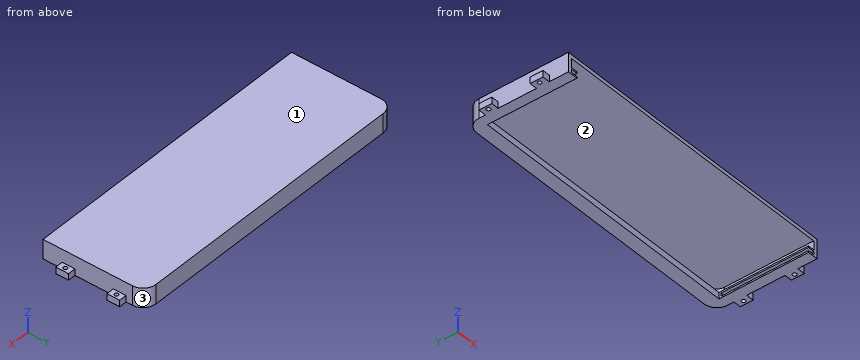
```python
from build123d import *

# Parameters (mm, degrees)
BOSS_EXTRU_1_DEPTH      = 15
COQUE1_T                = -3
ESQUISSE3_W             = 228
ESQUISSE3_H             = 3
ENL_V_MAT_EXTRU_2_DEPTH = 12
BOSS_EXTRU_3_DEPTH      = 5
BOSS_EXTRU_4_DEPTH      = 5
ESQUISSE2_W             = 6
ESQUISSE2_H             = 10
ESQUISSE2_R             = 1.5
BOSS_EXTRU_6_DEPTH      = 5


with BuildPart() as part:
    # Esquisse1 → Boss.-Extru.1 (new body)
    with BuildSketch(Plane.XY):
        with BuildLine():
            Line((-107, 40), (107, 40))
            ThreePointArc((107, 40), (114.071067812, 37.071067812), (117, 30))
            Line((117, 30), (117, -40))
            Line((117, -40), (-117, -40))
            Line((-117, -40), (-117, 30))
            ThreePointArc((-117, 30), (-114.071067812, 37.071067812), (-107, 40))
        make_face()
    extrude(amount=BOSS_EXTRU_1_DEPTH)

    # Coque1
    coque1_openings = [part.faces().sort_by_distance(p)[0] for p in [
        (0, -0.086787891, 0),
    ]]
    offset(amount=COQUE1_T, openings=coque1_openings, kind=Kind.INTERSECTION)

    # Esquisse3 → Enlèv. mat.-Extru.2 (cut)
    with BuildSketch(Plane(origin=(0, 0, 0), x_dir=(-1, 0, 0), z_dir=(0, 0, -1))):
        with Locations((0, -38.5)):
            Rectangle(ESQUISSE3_W, ESQUISSE3_H)
    extrude(amount=-ENL_V_MAT_EXTRU_2_DEPTH, mode=Mode.SUBTRACT)

    # Esquisse4 → Boss.-Extru.3 (add)
    with BuildSketch(Plane.ZY.offset(-114)):
        Polygon((0, -40), (0, 30), (5, 30), (5, -40), (3.75, -40), (3.75, 28.5), (1.25, 28.5), (1.25, -40), align=None)
    boss_extru_3 = extrude(amount=BOSS_EXTRU_3_DEPTH)

    # Symétrie1: Boss.-Extru.3 across plane
    add(boss_extru_3.mirror(Plane(origin=(0, 0, 0), x_dir=(0, 0, 1), z_dir=(1, 0, 0))))

    # Esquisse5 → Boss.-Extru.4 (add)
    with BuildSketch(Plane(origin=(0, 0, 0), x_dir=(-1, 0, 0), z_dir=(0, 0, -1))):
        with BuildLine():
            Line((-107, 37), (107, 37))
            ThreePointArc((107, 37), (111.949747468, 34.949747468), (114, 30))
            Line((114, 30), (-114, 30))
            ThreePointArc((-114, 30), (-111.949747468, 34.949747468), (-107, 37))
        make_face()
    extrude(amount=-BOSS_EXTRU_4_DEPTH)

    # Esquisse2 → Boss.-Extru.6 (add)
    # profile 1 of 4: a face of its own
    with BuildSketch(Plane(origin=(0, 0, 0), x_dir=(-1, 0, 0), z_dir=(0, 0, -1))):
        with Locations((-120, -20)):
            Rectangle(ESQUISSE2_W, ESQUISSE2_H)
        with Locations((-120, -20)):
            Circle(ESQUISSE2_R, mode=Mode.SUBTRACT)
    # profile 2 of 4: a face of its own
    with BuildSketch(Plane(origin=(0, 0, 0), x_dir=(-1, 0, 0), z_dir=(0, 0, -1))):
        with Locations((-120, 20)):
            Rectangle(ESQUISSE2_W, ESQUISSE2_H)
        with Locations((-120, 20)):
            Circle(ESQUISSE2_R, mode=Mode.SUBTRACT)
    # profile 3 of 4: a face of its own
    with BuildSketch(Plane(origin=(0, 0, 0), x_dir=(-1, 0, 0), z_dir=(0, 0, -1))):
        with Locations((120, 20)):
            Rectangle(ESQUISSE2_W, ESQUISSE2_H)
        with Locations((120, 20)):
            Circle(ESQUISSE2_R, mode=Mode.SUBTRACT)
    # profile 4 of 4: a face of its own
    with BuildSketch(Plane(origin=(0, 0, 0), x_dir=(-1, 0, 0), z_dir=(0, 0, -1))):
        with Locations((120, -20)):
            Rectangle(ESQUISSE2_W, ESQUISSE2_H)
        with Locations((120, -20)):
            Circle(ESQUISSE2_R, mode=Mode.SUBTRACT)
    extrude(amount=-BOSS_EXTRU_6_DEPTH)


solid = part.part
```
The listing builds one solid part. Answer for the finished solid, in the listing's coordinates (mm). Face numbers are marked on the shaded views. Coordinates: 2 decimals unless noted, no trailing zeros. Write each loop counter-clockwise with the first axis right and the second up, starting at its lowest first coordinate (ties: lowest second). Pieces come first, ordered by that corner, then holes.
Q1. Section A-A, the plane x = -39.5 is taken. Write down the section's boundary in (y, z), then the cut area to 3 significant figures.
Returned:
outline: (-40, 12) - (37, 12) - (37, 5) - (30, 5) - (30, 0) - (40, 0) - (40, 15) - (-40, 15) - close
area: 311 mm2
Q2. Given P1, Ø1.5, axis at y = 9.5, z = 7, coming from the +X side; P2, Ø6, axis at x = -26.5, z = 5.5, coming from the -Y side; P3, Ø1.5, axis at x = 120.5, z = 3, coming from the -Y side; P4, Ø1.8, axis at x = -120, y = -20, coming from the -Z side, each flat-ended and moving along its own axis, determine where each tip first touches the part or whether it passes through.
Returned:
P1: stops at x = 117
P2: stops at y = 30
P3: stops at y = -25
P4: passes through
Q3. The mould has two halves that part along X. Classify the marked faces 1, 2 and 3: released by +X, released by -X, zero draft, split by the parting line, or undercut.
Returned:
face 1: zero draft
face 2: undercut
face 3: released by +X
Q4. Section B-B, the plane z = 8.5 is taken. Write down the section's boundary in (x, y), then the cut area to 3 significant figures.
Returned:
outline: (-117, -40) - (-114, -40) - (-114, 30) arc R7 cw to (-107, 37) - (107, 37) arc R7 cw to (114, 30) - (114, -40) - (117, -40) - (117, 30) arc R10 ccw to (107, 40) - (-107, 40) arc R10 ccw to (-117, 30) - close
area: 1,140 mm2
Q5. Section C-C, the plane y = 5 is taken. Write down the section's boundary in (x, z), then the cut area to 3 significant figures.
Returned:
outline: (-117, 0) - (-109, 0) - (-109, 1.25) - (-114, 1.25) - (-114, 3.75) - (-109, 3.75) - (-109, 5) - (-114, 5) - (-114, 12) - (114, 12) - (114, 5) - (109, 5) - (109, 3.75) - (114, 3.75) - (114, 1.25) - (109, 1.25) - (109, 0) - (117, 0) - (117, 15) - (-117, 15) - close
area: 799 mm2
Q6. Find the intervals of material crossed by line 1 along Z through (x, y) = (-109.5, 12.5); line 2 along Y through (x, z) = (-120, 3.15); line 3 along X through (y, z) = (-2, 11.5), in increasing order.
Returned:
line 1: z = 0 to 1.25, 3.75 to 5, 12 to 15
line 2: y = -25 to -21.5, -18.5 to -15, 15 to 18.5, 21.5 to 25
line 3: x = -117 to -114, 114 to 117
